The listing builds one solid part. Answer for the finished solid, in the listing's coordinates (mm). Face numbers are marked on the shaded views. Give positions to 0.01 mm unless a question says otherwise; leave off trailing zeros. Write each loop counter-clockwise with the first axis right and the second up, starting at its lowest first coordinate (ties: lowest second). Pieces come first, ordered by that corner, then holes. Notation, with made-up numbers: (-12.75, 67.25) -> (-8.75, 67.25) arc R6 cw to (-8.75, 76.25) -> close; hole circle Ø5 at (-26.5, -25.75). An arc over 180 degrees is marked (long way). One line per question, with ' | ' between items.
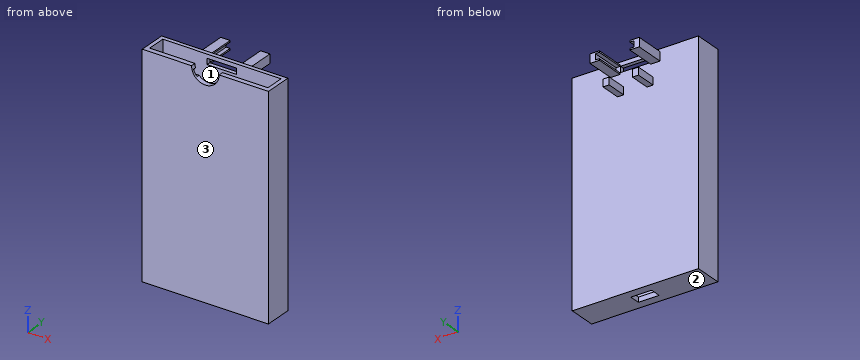
from build123d import *

# Parameters (mm, degrees)
ESQUISSE1_W                   = 128
ESQUISSE1_H                   = 28
ESQUISSE1_W_2                 = 120
ESQUISSE1_H_2                 = 19
CORPS_CASIER_DEPTH            = 220
PAROI_FOND_START              = -215
ESQUISSE2_W                   = 120
ESQUISSE2_H                   = 19
ESQUISSE2_W_2                 = 21
ESQUISSE2_H_2                 = 11
PAROI_FOND_DEPTH              = 5
ESQUISSE3_W                   = 6
ESQUISSE3_H                   = 6
ESQUISSE3_H_2                 = 4
FENTE_ET_ENCOCHE_VERROU_DEPTH = 15
ESQUISSE4_R                   = 14
ENCOCHE_PRISE_DOIGT_DEPTH     = 6
GLISSIERES_VERROU_START       = 28
GLISSIERES_VERROU_DEPTH       = 30
SUPPORTS_SERVO_SG90_START     = 28
ESQUISSE6_W                   = 6.2
ESQUISSE6_H                   = 7.5
SUPPORTS_SERVO_SG90_DEPTH     = 21.1


with BuildPart() as part:
    # Esquisse1 → Corps_casier (new body)
    with BuildSketch(Plane.XY):
        with Locations((0, 14)):
            Rectangle(ESQUISSE1_W, ESQUISSE1_H)
        with Locations((0, 14.5)):
            Rectangle(ESQUISSE1_W_2, ESQUISSE1_H_2, mode=Mode.SUBTRACT)
    extrude(amount=-CORPS_CASIER_DEPTH)

    # Esquisse2 → Paroi_fond (add)
    with BuildSketch(Plane.XY.offset(PAROI_FOND_START)):
        with Locations((0, 14.5)):
            Rectangle(ESQUISSE2_W, ESQUISSE2_H)
        with Locations((0, 14)):
            Rectangle(ESQUISSE2_W_2, ESQUISSE2_H_2, mode=Mode.SUBTRACT)
    extrude(amount=-PAROI_FOND_DEPTH)

    # Esquisse3 → Fente_et_encoche_verrou (cut, symmetric)
    with BuildSketch(Plane(origin=(0, 0, 0), x_dir=(0, 0, -1), z_dir=(1, 0, 0))):
        with Locations((7, 26)):
            Rectangle(ESQUISSE3_W, ESQUISSE3_H)
        with Locations((7, 4)):
            Rectangle(ESQUISSE3_W, ESQUISSE3_H_2)
    extrude(amount=FENTE_ET_ENCOCHE_VERROU_DEPTH, both=True, mode=Mode.SUBTRACT)

    # Esquisse4 → Encoche_prise_doigt (cut)
    with BuildSketch(Plane(origin=(0, 0, 0), x_dir=(1, 0, 0), z_dir=(0, 1, 0))):
        Circle(ESQUISSE4_R)
    extrude(amount=ENCOCHE_PRISE_DOIGT_DEPTH, mode=Mode.SUBTRACT)

    # Esquisse5 → Glissieres_verrou (add)
    with BuildSketch(Plane(origin=(0, 0, 0), x_dir=(1, 0, 0), z_dir=(0, 1, 0)).offset(GLISSIERES_VERROU_START)):
        Polygon((-25, 2.5), (-15.5, 2.5), (-15.5, 4), (-19.5, 4), (-19.5, 10), (-15.5, 10), (-15.5, 11.5), (-25, 11.5), align=None)
        Polygon((25, 2.5), (15.5, 2.5), (15.5, 4), (19.5, 4), (19.5, 10), (15.5, 10), (15.5, 11.5), (25, 11.5), align=None)
    extrude(amount=GLISSIERES_VERROU_DEPTH)

    # Esquisse6 → Supports_servo_SG90 (add)
    with BuildSketch(Plane(origin=(0, 0, 0), x_dir=(1, 0, 0), z_dir=(0, 1, 0)).offset(SUPPORTS_SERVO_SG90_START)):
        with Locations((-14.9, 28.25)):
            Rectangle(ESQUISSE6_W, ESQUISSE6_H)
        with Locations((14.9, 28.25)):
            Rectangle(ESQUISSE6_W, ESQUISSE6_H)
    extrude(amount=SUPPORTS_SERVO_SG90_DEPTH)


solid = part.part
Item 1: Find section C-C (z = -59.5). Write down the section's boundary in (x, y), then the cut area to 3 significant figures.
Answers below:
outline: (-64, 0) -> (64, 0) -> (64, 28) -> (-64, 28) -> close; hole (-60, 5) -> (60, 5) -> (60, 24) -> (-60, 24) -> close | area: 1,300 mm²
Item 2: Find section A-A (y = 41). Write down the section's boundary in (x, z), then the cut area to 3 significant figures.
Answers below:
outline: (-25, -11.5) -> (-15.5, -11.5) -> (-15.5, -10) -> (-19.5, -10) -> (-19.5, -4) -> (-15.5, -4) -> (-15.5, -2.5) -> (-25, -2.5) -> close; (-18, -32) -> (-11.8, -32) -> (-11.8, -24.5) -> (-18, -24.5) -> close; (11.8, -32) -> (18, -32) -> (18, -24.5) -> (11.8, -24.5) -> close; (15.5, -11.5) -> (25, -11.5) -> (25, -2.5) -> (15.5, -2.5) -> (15.5, -4) -> (19.5, -4) -> (19.5, -10) -> (15.5, -10) -> close | area: 216 mm²
Item 3: Flat-ended cylindrical pins translate along their axes: pin 1 (1 mm diameter, centred on x = -14.5, y = 21, fed in from +Z); pin 2 (1.9 mm diameter, centred on x = 13.5, y = 35, fed in from +Z); pin 3 (1.9 mm diameter, centred on x = -14, z = -29, fed in from +Y). Find the tip coordinate at first contact, or state that the pin passes through.
Answers below:
pin 1: z = -215 | pin 2: z = -24.5 | pin 3: y = 49.1
Item 4: Consider line 1 (Y direction, x = 23.5, z = -23); line 2 (X direction, y = 10, z = -110); line 3 (Z direction, x = -14, y = 20). Determine where each line is inside the solid, lowest interval first. Write a range as [from, to].
Answers below:
line 1: [0, 5], [24, 28] | line 2: [-64, -60], [60, 64] | line 3: [-220, -215]
Item 5: Determine the mould class of the marked faces 1, 2 and 3 for opening direction Y: pulls with the +Y half, pulls with the -Y half, needs draft (parallel to the pull), parting line crosses it, or undercut.
Answers below:
face 1: undercut | face 2: needs draft | face 3: pulls with the -Y half
Item 6: Find section B-B (x = 0). Write down the section's boundary in (y, z).
Answers below:
outline: (0, -220) -> (8.5, -220) -> (8.5, -215) -> (5, -215) -> (5, -14) -> (0, -14) -> close; (19.5, -220) -> (28, -220) -> (28, -10) -> (24, -10) -> (24, -215) -> (19.5, -215) -> close; (24, -4) -> (28, -4) -> (28, 0) -> (24, 0) -> close
Item 7: Find section D-D (x = 31.5). Write down the section's boundary in (y, z), then the cut area to 4 significant figures.
Answers below:
outline: (0, -220) -> (28, -220) -> (28, 0) -> (24, 0) -> (24, -215) -> (5, -215) -> (5, 0) -> (0, 0) -> close | area: 2,075 mm²
